```python
from build123d import *

# Parameters (mm, degrees)
F0_W = 1.0458609164
F0_H = 5.7817278951


with BuildPart() as f1:
    # F0 (on Front) → F1 (revolve)
    with BuildSketch(Plane.XZ):
        with Locations((-41.4770695418, -8.8908639476)):
            Rectangle(F0_W, F0_H)
        Polygon((0, -6), (0, -5), (-42, -5), (-42, -6), (-40.9541390836, -6), align=None)
        with Locations((41.4770695418, -8.8908639476)):
            Rectangle(F0_W, F0_H)
        Polygon((42, -5), (0, -5), (0, -6), (40.9541390836, -6), (42, -6), align=None)
    revolve(axis=Axis((-5.3423042409, 0, 0), (-1, 0, 0)))


solid = f1.part
```
Part model, mm, in its own coordinate system. A direction names the side the tool comes from. Round coordinates to 2 decimals unless told otherwise and drop trailing zeros. Write each loop counter-clockwise with the first axis right and the second up, starting at its lowest first coordinate (ties: lowest second). Pieces come first, ordered by that corner, then holes. Notation, with made-up numbers: (-29, 28) -> (-15, 28) arc R24 ccw to (-15, 57) -> close; hole circle Ø2 at (49.5, 40). An arc over 180 degrees is marked (long way). Return JSON: item names as keys, results as strings. Group by question number.
Q1. Probe L1, parallel to Y at x = -12.5, z = 0; L2, parallel to X at y = 5, z = 8.75. List the from-to ranges inside material, lowest first. Write a range as [from, to].
Q2. Saw through at A-A on y = 0. Write the cut outline in (x, z), plus the area to 3 significant figures.
Q3. Which spindle directions (+Z, -Z, +X, -X, +Y, -Y) get a long thin tool onto all of the face, cutting with end or side? Do faces 5 (the flat face through (-40.954, 5, -5)), 6 (the cylindrical face through (-41.47, -7.963, 8.684)). Say none if no direction does.
Q4. Saw through at D-D on z = 7.5. Write the cut outline in (x, y), plus the area to 3 significant figures.
Q5. Mould opens along X. For faces 1 (the flat face through (40.954, 5, -5)), 2 (the cylindrical face through (-0.59, 4.88, 1.08)), 3 (the flat face through (-42, 2, 5)), 4 (the flat face through (42, 2, -5)) say: pulls with the +X half, pulls with the -X half, needs draft (parallel to the pull), parting line crosses it, or undercut.
Q6. Saw through at C-C on x = 36.5. Write the cut outline in (y, z).
Q7. Pin check, flat tips, straight feed: pin 1 (12 mm diameter, centred on x = -22.5, z = 8.5, fed in from -Y); pin 2 (4 mm diameter, centred on x = -21, y = -1.5, fed in from -Z); pin 3 (6 mm diameter, centred on x = -3, z = 5.5, fed in from +Y). Stop position of each tip, or through.
Answer:
{
 "1": {"L1": "[-6, -5], [5, 6]", "L2": "[-42, -40.95], [40.95, 42]"},
 "2": {"outline": "(-42, -11.78) -> (-40.95, -11.78) -> (-40.95, -6) -> (40.95, -6) -> (40.95, -11.78) -> (42, -11.78) -> (42, -5) -> (-42, -5) -> close; (-42, 5) -> (42, 5) -> (42, 11.78) -> (40.95, 11.78) -> (40.95, 6) -> (-40.95, 6) -> (-40.95, 11.78) -> (-42, 11.78) -> close", "area": "192 mm2"},
 "3": {"face 5": "none", "face 6": "+X, -X"},
 "4": {"outline": "(-42, -9.09) -> (-40.95, -9.09) -> (-40.95, 9.09) -> (-42, 9.09) -> close; (40.95, -9.09) -> (42, -9.09) -> (42, 9.09) -> (40.95, 9.09) -> close", "area": "38.0 mm2"},
 "5": {"face 1": "undercut", "face 2": "needs draft", "face 3": "pulls with the -X half", "face 4": "pulls with the +X half"},
 "6": {"outline": "circle Ø12 at (0, 0); hole circle Ø10 at (0, 0)"},
 "7": {"pin 1": "y = -5.45", "pin 2": "z = -6", "pin 3": "y = 5.45"}
}
